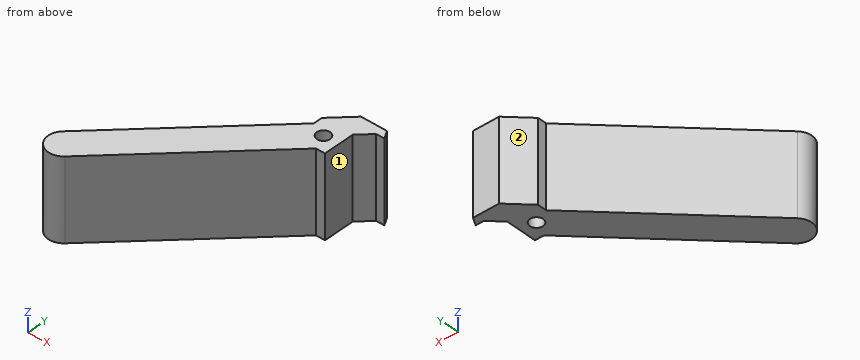
from build123d import *

# Parameters (mm, degrees)
BOSS_EXTRUDE1_DEPTH      = 9.9
BOSS_EXTRUDE1_DEPTH_BACK = 9.9
SKETCH1_W                = 7.5
SKETCH1_H                = 7.5
SKETCH1_R                = 1.6
BOSS_EXTRUDE2_DEPTH      = 19.8
BOSS_EXTRUDE3_START      = -19.8
SKETCH3_R                = 1.6
BOSS_EXTRUDE3_DEPTH      = 19.8


with BuildPart() as part:
    # Sketch1 → Boss-Extrude1 (new, two sides: drawn at the far end of the back side and taken through both)
    with BuildSketch(Plane.XY.offset(-BOSS_EXTRUDE1_DEPTH_BACK)):
        Rectangle(SKETCH1_W, SKETCH1_H)
        Circle(SKETCH1_R, mode=Mode.SUBTRACT)
    extrude(amount=BOSS_EXTRUDE1_DEPTH + BOSS_EXTRUDE1_DEPTH_BACK)

    # Sketch2 → Boss-Extrude2 (add)
    with BuildSketch(Plane.XY.offset(9.9)):
        Polygon((3.75, 3.75), (6.75, 6.75), (8.75, 6.75), (7.595299462, 8.75), (1.25, 8.75), (-3.75, 3.75), align=None)
    extrude(amount=-BOSS_EXTRUDE2_DEPTH)

    # Sketch3 → Boss-Extrude3 (add)
    with BuildSketch(Plane.XY.offset(9.9).offset(BOSS_EXTRUDE3_START)):
        with BuildLine():
            Line((2.651650429, -2.651650429), (-30.646899338, -35.950200197))
            ThreePointArc((-30.646899338, -35.950200197), (-35.950200197, -35.950200197), (-35.950200197, -30.646899338))
            Line((-35.950200197, -30.646899338), (-2.651650429, 2.651650429))
            ThreePointArc((-2.651650429, 2.651650429), (2.651650429, 2.651650429), (2.651650429, -2.651650429))
        make_face()
        Circle(SKETCH3_R, mode=Mode.SUBTRACT)
    extrude(amount=BOSS_EXTRUDE3_DEPTH)


solid = part.part
Model file for the job. Use its own axes, mm. Face numbers are marked on the shaded views. A direction names the side the tool comes from. Give positions to 0.01 mm unless a question says otherwise; leave off trailing zeros. Order: outer loops, then holes, each group sorted by start corner. A loop starts at its lowest first (then second) coordinate and runs counter-clockwise, first axis right, second up. Notation, with made-up numbers: M -8,-23 L 7,-23 A15 cw 7,-3 Z; hole C 21,56.5 d11. An arc over 180 degrees is marked long. Put each result on its own line as item: value. Start each with the question number.
(1) Tool access for the marked faces 1 and 2: list every direction of +Z, -Z, +X, -X, +Y, -Y with a clear straight run to the whole face (end or side of a thin tool).
(2) Band-saw the part on B-B on y = 0. Give the cut face in (x, z), then the cut area to 3 significant figures.
(3) Drill centre lines: L1, parallel to Y at x = 0, z = -4.75; L2, parallel to X at y = -5, z = 2; L3, parallel to X at y = -20.5, z = 4. Where is each one in solid material? Low to high. Write a range as [from, to].
(4) Pin check, flat tips, straight feed: pin 1 Ø8 at (y, z) = (0.5, 1) entering from +X; pin 2 Ø1 at (x, z) = (-27, 1) entering from +Y; pin 3 Ø10 at (y, z) = (0.5, -6) entering from +X; pin 4 Ø2.5 at (x, y) = (0, 0) entering from -Z. Stop position of each tip, or through.
(5) Band-saw the part on A-A on z = -4.5. Give the cut face in (x, y), then the cut area to 3 significant figures.
(6) Band-saw the part on D-D on x = -31.5. Give the cut face in (y, z), then the cut area to 3 significant figures.
(7) Band-saw the part on C-C on x = 0. Give the cut face in (y, z).
Results below:
1. face 1: +Z, -Z, +X, -Y
1. face 2: +Z, -Z, -X, +Y
2. outline: M -5.3,-9.9 L -1.6,-9.9 L -1.6,9.9 L -5.3,9.9 Z; M 1.6,-9.9 L 3.75,-9.9 L 3.75,9.9 L 1.6,9.9 Z
2. area: 116 mm2
3. L1: y = [-5.3, -1.6], [1.6, 7.5]
3. L2: x = [-10.3, 0.3]
3. L3: x = [-25.8, -15.2]
4. pin 1: stops at x = 4.5
4. pin 2: stops at y = -21.2
4. pin 3: stops at x = 5.5
4. pin 4: passes through
5. outline: M -35.95,-30.65 A3.75 ccw -30.65,-35.95 L 1.55,-3.75 L 3.75,-3.75 L 3.75,3.75 L 6.75,6.75 L 8.75,6.75 L 7.6,8.75 L 1.25,8.75 L -3.75,3.75 L -3.75,1.55 Z; hole C 0,0 d3.2
5. area: 436 mm2
6. outline: M -36.59,-9.9 L -26.2,-9.9 L -26.2,9.9 L -36.59,9.9 Z
6. area: 206 mm2
7. outline: M -5.3,-9.9 L -1.6,-9.9 L -1.6,9.9 L -5.3,9.9 Z; M 1.6,-9.9 L 7.5,-9.9 L 7.5,9.9 L 1.6,9.9 Z
